Could you check a few things on this drawing? It's one solid part, dimensions in mm from its lowest x, y, z. A direction names the side the tool comes from. Coordinates: 2 decimals unless noted, no trailing zeros. Order: outer loops, then holes, each group sorted by start corner. A loop starts at its lowest first (then second) coordinate and runs counter-clockwise, first axis right, second up. Notation, with made-up numbers: (40, 30.5) - (58, 30.5) arc R26 cw to (58, 58.5) - close; hole circle Ø9 at (-31, 51.25). An arc over 180 degrees is marked (long way). Answer in a Markdown table with one row per item. Add a question column.
Item 1: Will these pins go through, and if not, where does the flat tip stop? pin 1 Ø5 at (x, y) = (19.5, 12.5) entering from -Z; pin 2 Ø1 at (y, z) = (23, 1.5) entering from +X (1 decimal); pin 3 Ø1 at (y, z) = (3, 3.5) entering from +X.
Item 2: I want a section at B-B (y = 14). Please give me the cut outline in (x, z).
Item 3: If I drill on line 1 along Y through (x, z) = (14, 1.05); line 2 along Z through (x, y) = (9.25, 13.25); line 3 along X through (y, z) = (14, 1.15), over which ranges is the centre line in solid material (lowest first)? Write a range as from..to.
Item 4: I want a section at D-D (x = 9.5). Please give me the cut outline in (y, z).
Item 5: Thinking about a two-plate mould opening in X: for the marked faces 1, 2 and 3, which applies, +X half, -X half, draft (parallel to the pull), parting line (faces both ways), or undercut?
Item 6: I want a section at A-A (x = 14). Please give me the cut outline in (y, z).
Item 7: On a 3-axis mill with a long thin cutter (end or side, diameter ignored), from which of +Z, -Z, +X, -X, +Y, -Y can I reach the whole of each face in a straight line? I mean the marked faces 4 and 5. Say none if no direction works.
Item 8: I want a section at C-C (z = 1.8). Please give me the cut outline in (x, y).
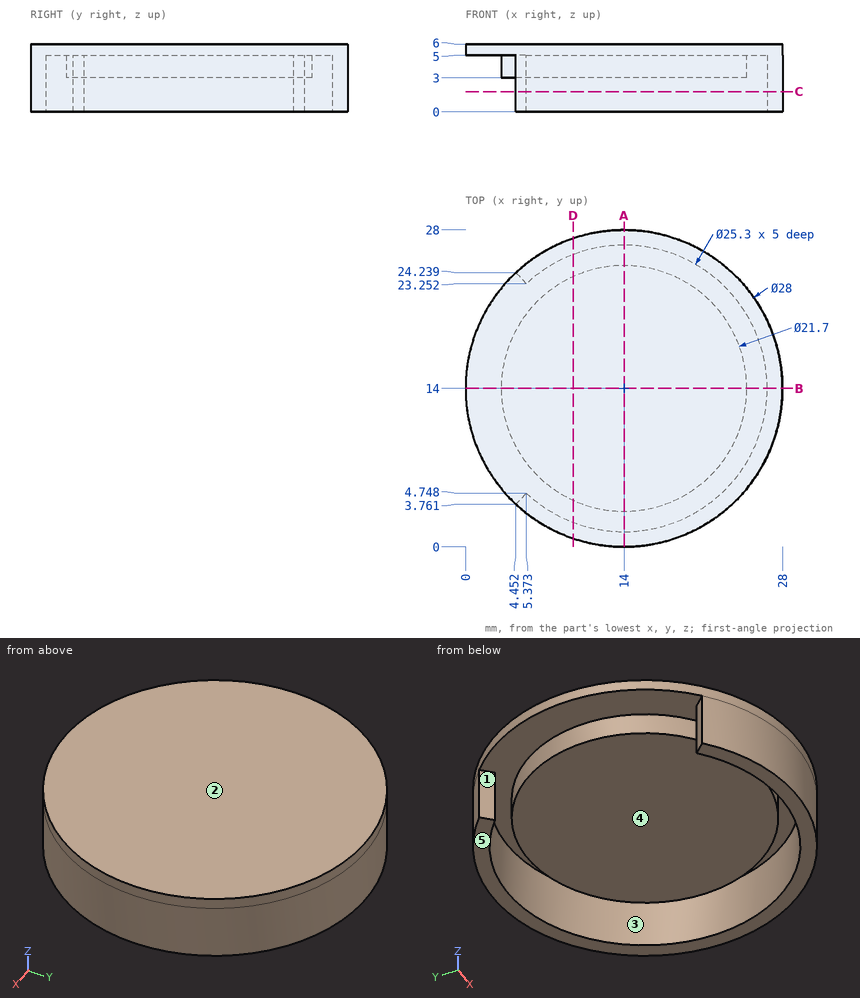
Values follow:
| question | item | result |
|---|---|---|
| 1 | pin 1 | stops at z = 3 |
| 1 | pin 2 | stops at x = 25.1 |
| 1 | pin 3 | stops at x = 23.26 |
| 2 | outline | (0, 5) - (3.15, 5) - (3.15, 3) - (24.85, 3) - (24.85, 5) - (26.65, 5) - (26.65, 0) - (28, 0) - (28, 6) - (0, 6) - close |
| 3 | line 1 | y = 0..1.35, 26.65..28 |
| 3 | line 2 | z = 3..6 |
| 3 | line 3 | x = 26.65..28 |
| 4 | outline | (0.74, 0) - (2.18, 0) - (2.18, 5) - (4.13, 5) - (4.13, 3) - (23.87, 3) - (23.87, 5) - (25.82, 5) - (25.82, 0) - (27.26, 0) - (27.26, 6) - (0.74, 6) - close |
| 5 | face 1 | -X half |
| 5 | face 2 | draft |
| 5 | face 3 | undercut |
| 6 | outline | (0, 0) - (1.35, 0) - (1.35, 5) - (3.15, 5) - (3.15, 3) - (24.85, 3) - (24.85, 5) - (26.65, 5) - (26.65, 0) - (28, 0) - (28, 6) - (0, 6) - close |
| 7 | face 4 | -Z |
| 7 | face 5 | -Z, +X, -X, +Y, -Y |
| 8 | outline | (4.45, 3.76) arc R14 ccw (long way) to (4.45, 24.24) - (5.37, 23.25) arc R12.65 cw (long way) to (5.37, 4.75) - close |
